Geometry: final body of the model. Coordinates: model frame, mm. Face numbers are marked on the shaded views. Coordinates: 2 decimals unless noted, no trailing zeros. Loops run counter-clockwise (first coordinate to the right, second up) from the corner with the lowest first, then second, coordinate; pieces in that order, holes last. Notation, with made-up numbers: (-16, 63.5) -> (30, 63.5) arc R18 cw to (30, 96.5) -> close; hole circle Ø2 at (-20.5, 67). An arc over 180 degrees is marked (long way). One line per item, written item: value. Start each with the question number.
Autodesk Inventor part; units mm, degrees
ref_plane "YZ Plane" through (0, 0, 0) normal (1, 0, 0) x (0, 1, 0)
ref_plane "XZ Plane" through (0, 0, 0) normal (0, 1, 0) x (-1, 0, 0)
ref_plane "XY Plane" through (0, 0, 0) normal (0, 0, 1) x (1, 0, 0)
sketch "Sketch1" plane through (0, 0, 0) normal (0, 1, 0) x (-1, 0, 0)
  line L0 (0, 0) -> (15, 0)
  line L1 (15, 0) -> (15, -2.5)
  line L2 (15, -2.5) -> (13.25, -2.5)
  line L3 (13.25, -2.5) -> (13.25, -4.5)
  line L4 (13.25, -4.5) -> (15, -4.5)
  line L5 (15, -4.5) -> (15, -7.5)
  line L6 (15, -7.5) -> (13.25, -7.5)
  line L7 (13.25, -7.5) -> (13.25, -9.5)
  line L8 (13.25, -9.5) -> (15, -9.5)
  line L9 (15, -9.5) -> (15, -12)
  line L10 (15, -12) -> (0, -12)
  line L11 (0, -12) -> (0, 0)
  dimension "d0" = 2.5
  dimension "d2" = 2.5
  dimension "d3" = 2
  dimension "d4" = 2
  dimension "d7" = 12
  dimension "d8" = 26.5
  dimension "d9" = 30
revolve "Revolution1" add sketch "Sketch1" angle 360 about axis through (0, 0, -12) along (0, 0, 1)
sketch "Sketch2" plane through (0, 0, -12) normal (0, 0, -1) x (-1, 0, 0)
  circle A0 centre (0, 0) radius 15
  point P0 (0, 0)
hole "Hole1" at (0, 0, -12) direction (0, 0, 1) diameter 6.647 end through all counterbore diameter 9 counterbore depth 5
properties part number "2021"
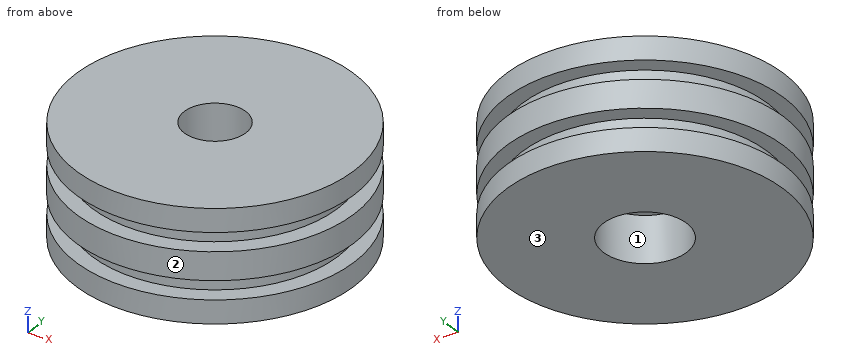
1. Draft query along X for the marked faces 1, 2 and 3. Return one class per face: released by +X, released by -X, zero draft, split by the parting line, or undercut.
2. Line query: L1, parallel to Z at x = 13.25, y = -3; L2, parallel to Y at x = 0, z = -5.5; L3, parallel to Y at x = 0, z = -10.05. Output: solid intervals per line, ascending. Write a range as [from, to].
3. Section D-D on y = -7.75. Return the cut outline in (x, z), plus the area to 3 significant figures.
4. Section C-C on z = -1.5. Return the cut outline in (x, y).
5. Section A-A on x = 0. Return the cut outline in (y, z), plus the area to 3 significant figures.
6. Pin query (flat end, axial travel): pin 1 Ø5 at (x, z) = (-5.5, -9) entering from +Y; pin 2 Ø2 at (y, z) = (-2.5, -9) entering from +X; pin 3 Ø6 at (x, z) = (-4, -2.5) entering from +Y. Return the tip coordinate at first contact, or that it passes through.
Checks:
1. face 1: undercut
1. face 2: split by the parting line
1. face 3: zero draft
2. L1: [-12, -9.5], [-7.5, -4.5], [-2.5, 0]
2. L2: [-15, -3.32], [3.32, 15]
2. L3: [-15, -4.5], [4.5, 15]
3. outline: (-12.84, -12) -> (12.84, -12) -> (12.84, -9.5) -> (10.75, -9.5) -> (10.75, -7.5) -> (12.84, -7.5) -> (12.84, -4.5) -> (10.75, -4.5) -> (10.75, -2.5) -> (12.84, -2.5) -> (12.84, 0) -> (-12.84, 0) -> (-12.84, -2.5) -> (-10.75, -2.5) -> (-10.75, -4.5) -> (-12.84, -4.5) -> (-12.84, -7.5) -> (-10.75, -7.5) -> (-10.75, -9.5) -> (-12.84, -9.5) -> close
3. area: 291 mm²
4. outline: circle Ø30 at (0, 0); hole circle Ø6.65 at (0, 0)
5. outline: (-15, -12) -> (-4.5, -12) -> (-4.5, -7) -> (-3.32, -7) -> (-3.32, 0) -> (-15, 0) -> (-15, -2.5) -> (-13.25, -2.5) -> (-13.25, -4.5) -> (-15, -4.5) -> (-15, -7.5) -> (-13.25, -7.5) -> (-13.25, -9.5) -> (-15, -9.5) -> close; (3.32, -7) -> (4.5, -7) -> (4.5, -12) -> (15, -12) -> (15, -9.5) -> (13.25, -9.5) -> (13.25, -7.5) -> (15, -7.5) -> (15, -4.5) -> (13.25, -4.5) -> (13.25, -2.5) -> (15, -2.5) -> (15, 0) -> (3.32, 0) -> close
5. area: 254 mm²
6. pin 1: y = 14.69
6. pin 2: x = 14.91
6. pin 3: y = 14.97
